Study the drawing (mm; zero at the part's minimum x, y, z) and answer. A direction names the side the tool comes from. Round coordinates to 2 decimals unless told otherwise and drop trailing zeros. Write each loop counter-clockwise with the first axis right and the second up, starting at its lowest first coordinate (ties: lowest second). Pieces come first, ordered by that corner, then holes.
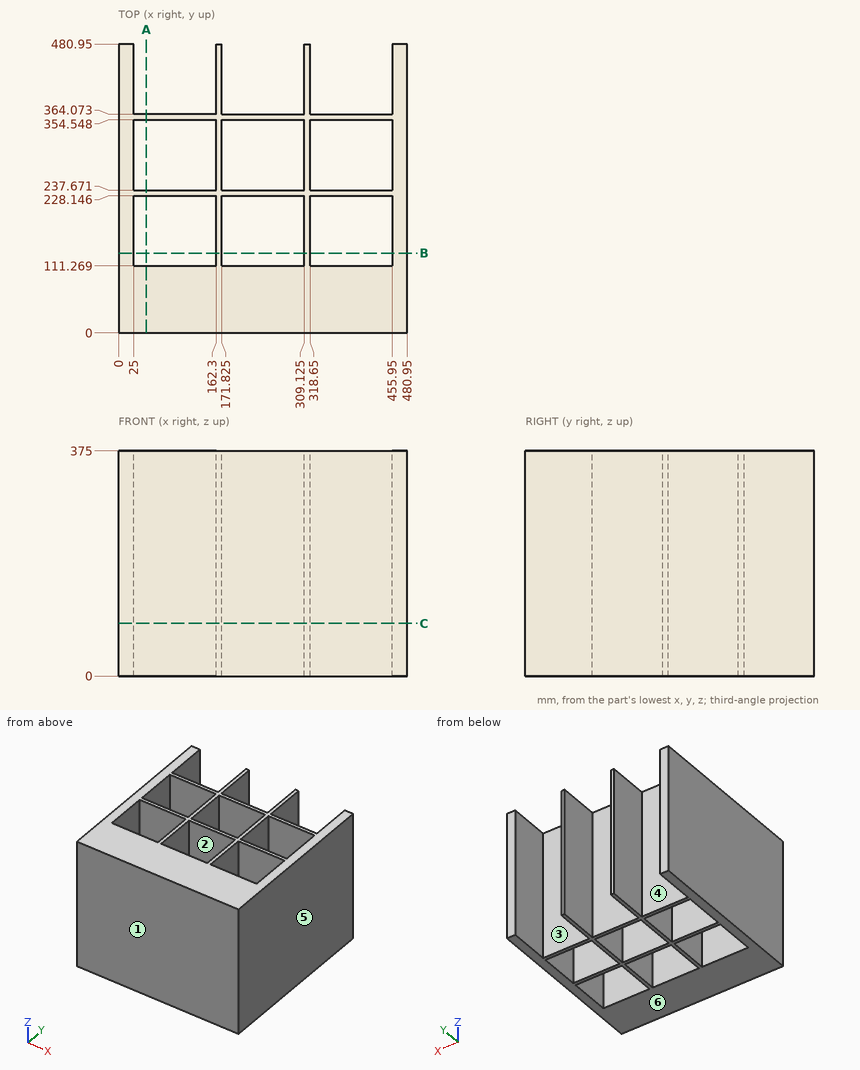
1. Straight lines are drawn through the part: line 1 along Y through (x, z) = (211, 62); line 2 along X through (y, z) = (296, 214) (3 decimals). For each, find the intervals that lie inside material, in ascending order.
Geometry says:
line 1: y = 0 to 111.27, 228.15 to 237.67, 354.55 to 364.07
line 2: x = 0 to 25, 162.3 to 171.825, 309.125 to 318.65, 455.95 to 480.95
2. A tool of negligible diameter and unlimited length cuts with its end or side. For the marked faces 1, 2 and 3, from which of +Z, -Z, +X, -X, +Y, -Y can it reach the whole face along a straight path? Write none if from no direction.
Geometry says:
face 1: +Z, -Z, +X, -X, -Y
face 2: +Z, -Z
face 3: +Z, -Z, +Y
3. For a pull along X with two mould halves and no side action, classify the marked faces 4, 5 and 6 as released by +X, released by -X, zero draft, split by the parting line, or undercut.
Geometry says:
face 4: undercut
face 5: released by +X
face 6: zero draft
4. Section C-C on z = 87.5 is taken. Give the number of separate pieces and of enclosed holes in the cut face, plus the area to 3 significant figures.
Geometry says:
separate pieces: 1
enclosed holes: 6
area: 86,900 mm2
5. Section B-B on y = 132.5 is taken. Determine the outline of the cut face in (x, z) (3 decimals).
Geometry says:
outline: (0, 0) - (25, 0) - (25, 375) - (0, 375) - close; (162.3, 0) - (171.825, 0) - (171.825, 375) - (162.3, 375) - close; (309.125, 0) - (318.65, 0) - (318.65, 375) - (309.125, 375) - close; (455.95, 0) - (480.95, 0) - (480.95, 375) - (455.95, 375) - close
6. Given pin 1 (12 mm diameter, centred on x = 346, z = 310, fed in from +Y), flat-ended and moving along its own axis, determine where the tip first touches the part or whether it passes through.
Geometry says:
pin 1: stops at y = 364.07
7. Section A-A on x = 46 is taken. Determine the outline of the cut face in (y, z).
Geometry says:
outline: (0, 0) - (111.27, 0) - (111.27, 375) - (0, 375) - close; (228.15, 0) - (237.67, 0) - (237.67, 375) - (228.15, 375) - close; (354.55, 0) - (364.07, 0) - (364.07, 375) - (354.55, 375) - close
